Design review of the part built by this model. Coordinates are the model's own, in mm. A direction names the side the tool comes from. Give positions to 0.01 mm unless a question says otherwise; leave off trailing zeros. Loops run counter-clockwise (first coordinate to the right, second up) from the corner with the lowest first, then second, coordinate; pieces in that order, holes last. Notation, with made-up numbers: M 72.25,55 L 112.25,55 A35 ccw 112.25,92 Z; hole C 69.25,-29 d4. An arc over 180 degrees is marked long. Use CSV: the item, a comma, the result in double quotes.
from build123d import *

# Parameters (mm, degrees)
SKETCH1_R           = 1.6
BOSS_EXTRUDE1_DEPTH = 1.5
BOSS_EXTRUDE2_START = -4.9
BOSS_EXTRUDE2_DEPTH = 12.5


with BuildPart() as part:
    # Sketch1 → Boss-Extrude1 (new body)
    with BuildSketch(Plane.XY):
        with BuildLine():
            Line((-17.340213643, 2.359447139), (-21.303691048, 2.898749343))
            ThreePointArc((-21.303691048, 2.898749343), (-21.483854857, -0.833054911), (-21.015258676, -4.539702939))
            Line((-21.015258676, -4.539702939), (-16.893017252, -4.569022665))
            ThreePointArc((-16.893017252, -4.569022665), (-17.46366078, -1.127187719), (-17.340213643, 2.359447139))
        make_face()
        with Locations((-19.431785099, -0.930778688)):
            Circle(SKETCH1_R, mode=Mode.SUBTRACT)
        with BuildLine():
            ThreePointArc((-16.893017252, -4.569022665), (-7.75565719, -15.687567738), (6.62676566, -16.196789092))
            ThreePointArc((6.62676566, -16.196789092), (9.70800359, -14.560380019), (12.403398325, -12.345270754))
            ThreePointArc((12.403398325, -12.345270754), (15.300036009, -8.494639375), (17.036725037, -4))
            Line((17.036725037, -4), (28.5, -4))
            Line((28.5, -4), (28.5, 4))
            Line((28.5, 4), (17.036725037, 4))
            ThreePointArc((17.036725037, 4), (14.721119178, 9.462486468), (10.713447983, 13.837341952))
            ThreePointArc((10.713447983, 13.837341952), (7.75565719, 15.687567738), (4.489618927, 16.91429342))
            ThreePointArc((4.489618927, 16.91429342), (-9.70800359, 14.560380019), (-17.340213643, 2.359447139))
            ThreePointArc((-17.340213643, 2.359447139), (-17.46366078, -1.127187719), (-16.893017252, -4.569022665))
        make_face()
        with BuildLine():
            Line((10.713447983, 13.837341952), (13.162236094, 17.00016297))
            ThreePointArc((13.162236094, 17.00016297), (10.020480713, 19.022091533), (6.576131268, 20.46959935))
            Line((6.576131268, 20.46959935), (4.489618927, 16.91429342))
            ThreePointArc((4.489618927, 16.91429342), (7.75565719, 15.687567738), (10.713447983, 13.837341952))
        make_face()
        with Locations((8.909814561, 17.293808881)):
            Circle(SKETCH1_R, mode=Mode.SUBTRACT)
        with BuildLine():
            Line((6.62676566, -16.196789092), (8.141454954, -19.898912313))
            ThreePointArc((8.141454954, -19.898912313), (11.463374144, -18.189036622), (14.439127409, -15.929896411))
            Line((14.439127409, -15.929896411), (12.403398325, -12.345270754))
            ThreePointArc((12.403398325, -12.345270754), (9.70800359, -14.560380019), (6.62676566, -16.196789092))
        make_face()
        with Locations((10.521970538, -16.363030193)):
            Circle(SKETCH1_R, mode=Mode.SUBTRACT)
    extrude(amount=BOSS_EXTRUDE1_DEPTH)

    # Sketch2 → Boss-Extrude2 (add)
    with BuildSketch(Plane(origin=(28.5, 0, 0), x_dir=(0, 0, -1), z_dir=(1, 0, 0)).offset(BOSS_EXTRUDE2_START)):
        with BuildLine():
            ThreePointArc((6, -2.75), (3.25, 0), (6, 2.75))
            Line((6, 2.75), (0, 2.898749343))
            Line((0, 2.898749343), (0, -2.752957148))
            Line((0, -2.752957148), (6, -2.75))
        make_face()
    extrude(amount=-BOSS_EXTRUDE2_DEPTH)


solid = part.part
(1) The part is to be moulded in two halves that separate along X. For faces 1 (the flat face through (-19.294, 2.625, 0.74)), 2 (the flat face through (3, 1, 1.5)), 3 (the flat face through (11.921, 15.397, 0.74)), say which applies: released by +X, released by -X, zero draft, split by the parting line, or undercut.
A:
face 1,"undercut"
face 2,"zero draft"
face 3,"released by +X"
(2) We need section C-C on x = 2.5. State the section outline as (y, z) points, then the cut area to 3 significant figures.
A:
outline,"M -17.32,0 L 17.32,0 L 17.32,1.5 L -17.32,1.5 Z"
area,"52.0 mm²"
(3) Machinability: for faces 4 (the flat face through (23, 4, 1)), 5 (the flat face through (13.436, -14.163, 0.74)), 6 (the flat face through (23, -4, 1)), 7 (the flat face through (23.6, 0, -2)), 8 (the flat face through (7.374, -18.022, 0.74)), which of the approach directions +Z, -Z, +X, -X, +Y, -Y give a long, thin tool a straight path to every point of the face, cutting with its end or side? Answer none if there is none.
A:
face 4,"+Z, -Z, +X, +Y"
face 5,"+Z, -Z, +X"
face 6,"+Z, -Z, +X, -Y"
face 7,"-Z, +X, +Y, -Y"
face 8,"+Z, -Z, -Y"
(4) We need section B-B on y = 0. State the section outline as (x, z) points.
A:
outline,"M -21.5,0 L -20.73,0 L -20.73,1.5 L -21.5,1.5 Z; M -18.13,0 L 11.1,0 L 11.1,-3.25 L 23.6,-3.25 L 23.6,0 L 28.5,0 L 28.5,1.5 L -18.13,1.5 Z"
(5) We need section A-A on z = -4.25. State the section outline as (x, y) points.
A:
outline,"M 11.1,-2.75 L 23.6,-2.75 L 23.6,-2.12 L 11.1,-2.12 Z; M 11.1,2.12 L 23.6,2.12 L 23.6,2.79 L 11.1,2.79 Z"
(6) We need section D-D on y = -8.5. State the section outline as (x, z) points.
A:
outline,"M -15.3,0 L 15.3,0 L 15.3,1.5 L -15.3,1.5 Z"
(7) Wall thickness on line 1 along Y through (x, z) = (11.5, 1); line 2 along Z through (x, y) = (2.5, 4.5); line 3 along Y through (x, z) = (13.5, -4.25): over which ranges is each line inside the solid? List them lowest first. Write a range as [from, to].
A:
line 1,"[-18.17, -17.63], [-15.1, 13.19], [14.85, 18.17]"
line 2,"[0, 1.5]"
line 3,"[-2.75, -2.12], [2.12, 2.79]"
(8) Clearance check with flat-ended pins moving along their axes: P1, Ø4, axis at x = -19.43, y = -0.93, coming from the -Z side; P2, Ø1.7, axis at y = -1, z = -4, coming from the +X side; P3, Ø1.6, axis at x = 24.5, z = 0.5, coming from the +Y side; P4, Ø3, axis at x = 8.91, y = 17.29, coming from the -Z side. State where each tip first meets the part, or that it passes through.
A:
P1,"z = 0"
P2,"x = 23.6"
P3,"y = 4"
P4,"through"
